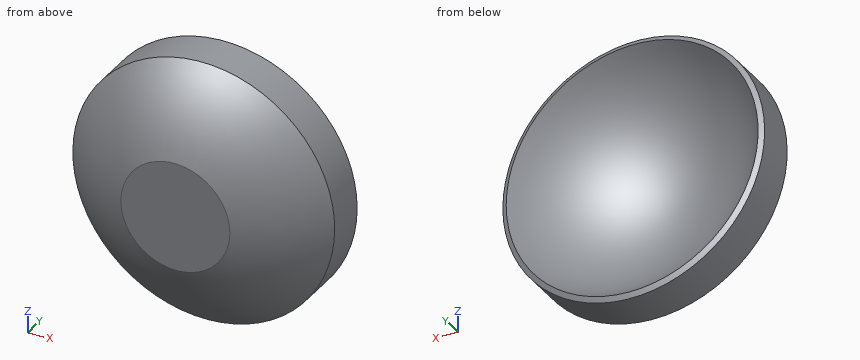
```python
from build123d import *

# Parameters (mm, degrees)
SKETCH_2_W               = 1.902691091
SKETCH_2_H               = 5.293337887
SKETCH_3_W               = 11.904020265
SKETCH_3_H               = 2.403246825
CUT_EXTRUDE_1_DEPTH      = 5.5
CUT_EXTRUDE_1_DEPTH_BACK = 5.5


with BuildPart() as part:
    # Эскиз1 one side → Повернуть1 (revolve)
    with BuildSketch(Plane.XY):
        with BuildLine():
            Line((0, 0), (0, -1))
            ThreePointArc((0, -1), (3, -0.196152423), (5.196152423, 2))
            Line((5.196152423, 2), (4.330127019, 2.5))
            ThreePointArc((4.330127019, 2.5), (2.5, 0.669872981), (0, 0))
        make_face()
    revolve(axis=Axis((0, 0, 0), (0, -1, 0)))

    # Эскиз2 → Вырез-Повернуть1 (revolve, cut)
    with BuildSketch(Plane.XY):
        with Locations((-5.451345546, 1.418725327)):
            Rectangle(SKETCH_2_W, SKETCH_2_H)
    revolve(axis=Axis((0, 0, 0), (0, 1, 0)), mode=Mode.SUBTRACT)

    # Эскиз3 → Вырез-Вытянуть1 (cut, two sides)
    with BuildSketch(Plane.XY) as cut_extrude_1_sk:
        with Locations((-0.172996367, -1.901623413)):
            Rectangle(SKETCH_3_W, SKETCH_3_H)
    extrude(amount=CUT_EXTRUDE_1_DEPTH, mode=Mode.SUBTRACT)
    extrude(cut_extrude_1_sk.sketch, amount=-CUT_EXTRUDE_1_DEPTH_BACK, mode=Mode.SUBTRACT)


solid = part.part
```
Input: part model. Units: mm. Frame: model coordinates. Coordinates: 2 decimals unless noted, no trailing zeros. Loops run counter-clockwise (first coordinate to the right, second up) from the corner with the lowest first, then second, coordinate; pieces in that order, holes last. Notation, with made-up numbers: M 37.25,0.25 L 79.25,0.25 A20 ccw 79.25,23.25 Z; hole C 82,-4 d1. An arc over 180 degrees is marked long. Answer in a Markdown table with one row per item.
1. Section B-B, the plane x = 0. Output: boundary loops of the cut face in (y, z).
Response:
| item | result |
|---|---|
| outline | M -0.7,-1.87 A6 ccw 1.03,-4.5 L 2.4,-4.5 L 2.5,-4.33 A5 cw 2.5,4.33 L 2.4,4.5 L 1.03,4.5 A6 ccw -0.7,1.87 Z |
2. Section D-D, the plane y = 1.35. Output: boundary loops of the cut face in (x, z), then the cut area to 3 significant figures.
Response:
| item | result |
|---|---|
| outline | C 0,0 d9; hole C 0,0 d6.83 |
| area | 26.9 mm2 |
3. Material intervals for line 1 (Z direction, x = 0.25, y = 2.2); line 2 (X direction, y = 1.6, z = 0.75); line 3 (X direction, y = 2, z = -3.5), sorted ascending.
Response:
| item | result |
|---|---|
| line 1 | z = -4.49 to -4.13, 4.13 to 4.49 |
| line 2 | x = -4.44 to -3.59, 3.59 to 4.44 |
| line 3 | x = -2.83 to -1.94, 1.94 to 2.83 |
4. Section A-A, the plane z = 0. Output: boundary loops of the cut face in (x, y), then the cut area to 3 significant figures.
Response:
| item | result |
|---|---|
| outline | M -4.5,1.03 A6 ccw -1.87,-0.7 L 1.87,-0.7 A6 ccw 4.5,1.03 L 4.5,2.4 L 4.33,2.5 A5 cw -4.33,2.5 L -4.5,2.4 Z |
| area | 9.76 mm2 |
5. First-contact query: pin 1 (1 mm diameter, centred on x = 3, z = -0.5, fed in from -Y). Flat tip, straight axial feed; report the tip coordinate or a pass-through.
Response:
| item | result |
|---|---|
| pin 1 | stops at y = -0.44 |
6. Section C-C, the plane y = 1.9. Output: boundary loops of the cut face in (x, z), then the cut area to 3 significant figures.
Response:
| item | result |
|---|---|
| outline | C 0,0 d9; hole C 0,0 d7.85 |
| area | 15.3 mm2 |
